Can you work these out from the model? Positions are in its coordinate system, mm. Face numbers are marked on the shaded views. Give positions to 0.01 mm unless a question says otherwise; leave off trailing zeros. Order: outer loops, then holes, each group sorted by start corner. A loop starts at its lowest first (then second) coordinate and runs counter-clockwise, first axis right, second up.
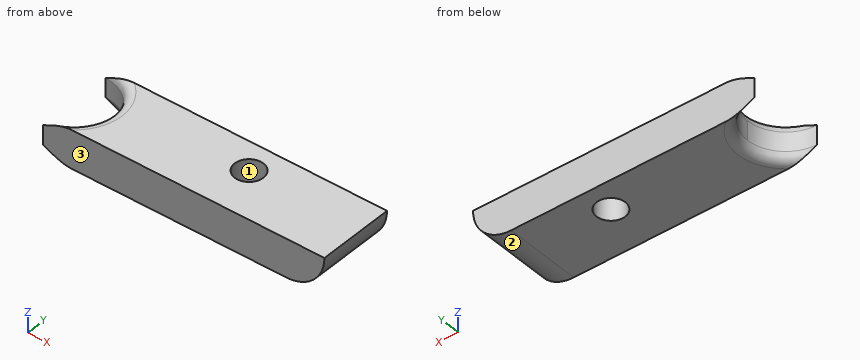
```python
from build123d import *

# Parameters (mm, degrees)
F0_R        = 1.5
F1_DEPTH    = 4
F2_T2_ANGLE = 301.9493341655
F2_T4_ANGLE = 301.9493341655
F3_R        = 3.99999


# Not quite as in the source:
# - a fillet or chamfer that OpenCascade refuses, or shapes differently, is made with other operations: its cross-section is extruded or revolved along the edge and cut away or added
# - a fillet or chamfer is up to 0.001 mm smaller than in the source, because OpenCascade refuses the exact size


with BuildPart() as f1:
    # F0 (on Top) → F1 (new body)
    with BuildSketch(Plane.XY):
        with BuildLine():
            ThreePointArc((0, 8), (2.8284271247, 6.8284271247), (4, 4))
            ThreePointArc((4, 4), (2.8284271247, 1.1715728753), (0, 0))
            Line((0, 0), (29.5, 0))
            Line((29.5, 0), (29.5, 8))
            Line((29.5, 8), (0, 8))
        make_face()
        with Locations((17.5, 5)):
            Circle(F0_R, mode=Mode.SUBTRACT)
    extrude(amount=F1_DEPTH)

    # F2: fillet of radius 1 on 2 edges, made by hand

    # F2_s1 → F2_t2 (revolve, cut)
    with BuildSketch(Plane(origin=(1.697032729, 3.0583382808, 0), x_dir=(0, 0, 1), z_dir=(-0.4851962797, -0.8744052666, 0))):
        with BuildLine():
            ThreePointArc((1, 5.9407851187), (0.2928932188, 6.2336783375), (0, 6.9407851187))
            Line((0, 6.9407851187), (0, 5.9407851187))
            Line((0, 5.9407851187), (1, 5.9407851187))
        make_face()
    revolve(axis=Axis((0, 4, 0), (0, 0, -1)), revolution_arc=F2_T2_ANGLE, mode=Mode.SUBTRACT)

    # F2_s3 → F2_t4 (revolve, cut)
    with BuildSketch(Plane(origin=(-1.697032729, 3.0583382808, 0), x_dir=(0, 0, 1), z_dir=(-0.4851962797, 0.8744052666, 0))):
        with BuildLine():
            ThreePointArc((3, -2.0592148813), (3.7071067812, -2.3521081002), (4, -3.0592148813))
            Line((4, -3.0592148813), (4, -2.0592148813))
            Line((4, -2.0592148813), (3, -2.0592148813))
        make_face()
    revolve(axis=Axis((0, 4, 4), (0, 0, 1)), revolution_arc=F2_T4_ANGLE, mode=Mode.SUBTRACT)

    # F3 (radius 4 in the source; OpenCascade refuses exactly that, so slightly less here)
    f3_edges = [f1.edges().sort_by_distance(p)[0] for p in [
        (29.5, 4, 0),
    ]]
    fillet(f3_edges, radius=F3_R)


solid = f1.part
```
1) We'd pull the mould along Y, two halves only. Please class the marked faces 1, 2 and 3: +Y half, -Y half, draft (parallel to the pull), parting line (faces both ways), or undercut.
2) Suppose I cut it at A-A (x = 17.5). Please give me the cut outline in (y, z), and give its area (3 significant figures).
3) Suppose I cut it at C-C (x = 27.25). Please give me the cut outline in (y, z), and give its area (3 significant figures).
4) Suppose I cut it at B-B (z = 2.3). Please give me the cut outline in (x, y), and give its area (3 significant figures).
5) If I drill on line 1 (Y direction, x = 17.5, z = 2.1); line 2 (Y direction, x = 1.75, z = 2.25); line 3 (X direction, y = 4.5, z = 3.4), over which ranges is the centre line in solid material (lowest first)?
Results:
1. face 1: undercut
1. face 2: draft
1. face 3: -Y half
2. outline: (0, 0) - (3.5, 0) - (3.5, 4) - (0, 4) - close; (6.5, 0) - (8, 0) - (8, 4) - (6.5, 4) - close
2. area: 20.0 mm2
3. outline: (0, 0.4) - (8, 0.4) - (8, 4) - (0, 4) - close
3. area: 28.8 mm2
4. outline: (0, 0) - (29.12, 0) - (29.12, 8) - (0, 8) arc R4 cw to start; hole circle Ø3 at (17.5, 5)
4. area: 201 mm2
5. line 1: y = 0 to 3.5, 6.5 to 8
5. line 2: y = 0 to 0.4, 7.6 to 8
5. line 3: x = 4.05 to 16.09, 18.91 to 29.45
